```python
from build123d import *

# Parameters (mm, degrees)
SKETCH1_R               = 6.35
SKETCH1_W               = 19.05
SKETCH1_H               = 25.985863096
EXTRUDE2_DEPTH          = 14.3002
SKETCH2_W               = 19.05
SKETCH2_H               = 69.85
EXTRUDE3_DEPTH          = 23.8252
CUT_EXTRUDE1_DEPTH      = 73.599512703
CUT_EXTRUDE1_DEPTH_BACK = 73.599512703
CUT_EXTRUDE2_START      = -19.05
CUT_EXTRUDE2_DEPTH      = 19.05
EXTRUDE4_DEPTH          = 19.05
EXTRUDE4_DEPTH_BACK     = 38.1
FILLET1_R               = 6.35


# Read off the part's stored shape, not the designer's step: Cut-Extrude2
with BuildPart() as part:
    # Sketch1 → Extrude2 (new body)
    # profile 1 of 2: a face of its own
    with BuildSketch(Plane(origin=(0, 0, 0), x_dir=(1, 0, 0), z_dir=(0, 1, 0))):
        Polygon((-44.03422619, -11.566071429), (-44.03422619, 14.419791667), (-72.60922619, 14.419791667), (-72.60922619, -42.730208333), (3.59077381, -42.730208333), (3.59077381, 14.419791667), (-24.98422619, 14.419791667), (-24.98422619, -11.566071429), align=None)
        with Locations(Location((-56.73422619, -26.855208333, 0), (0, 0, 270))):
            Circle(SKETCH1_R, mode=Mode.SUBTRACT)
        with Locations(Location((-12.28422619, -26.855208333, 0), (0, 0, 270))):
            Circle(SKETCH1_R, mode=Mode.SUBTRACT)
    # profile 2 of 2: a face of its own
    with BuildSketch(Plane(origin=(0, 0, 0), x_dir=(1, 0, 0), z_dir=(0, 1, 0))):
        with Locations((-34.50922619, 1.426860119)):
            Rectangle(SKETCH1_W, SKETCH1_H)
    extrude(amount=-EXTRUDE2_DEPTH)

    # Sketch2 → Extrude3 (add)
    with BuildSketch(Plane(origin=(0, 0, 0), x_dir=(-1, 0, 0), z_dir=(0, 1, 0))):
        with Locations((34.50922619, -14.419791667)):
            Rectangle(SKETCH2_W, SKETCH2_H)
    extrude(amount=EXTRUDE3_DEPTH)

    # Sketch3 → Cut-Extrude1 (cut, two sides: drawn at the far end of the back side and taken through both)
    with BuildSketch(Plane.ZY.offset(44.03422619).offset(-CUT_EXTRUDE1_DEPTH_BACK)):
        Polygon((20.505208333, 23.8252), (-14.419791667, 23.8252), (20.505208333, 0), align=None)
    extrude(amount=CUT_EXTRUDE1_DEPTH + CUT_EXTRUDE1_DEPTH_BACK, mode=Mode.SUBTRACT)

    # Cut-Extrude2 outline → Cut-Extrude2 (cut)
    with BuildSketch(Plane.ZY.offset(44.03422619).offset(CUT_EXTRUDE2_START)):
        Polygon((-49.344791667, 0), (-14.419791667, 0), (-49.344791667, 23.8252), align=None)
    extrude(amount=CUT_EXTRUDE2_DEPTH, mode=Mode.SUBTRACT)

    # Sketch5 → Extrude4 (add, two sides: drawn at the far end of the back side and taken through both)
    with BuildSketch(Plane(origin=(-24.98422619, 0, -14.419791667), x_dir=(0, 0, -1), z_dir=(1, 0, 0)).offset(-EXTRUDE4_DEPTH_BACK)):
        Polygon((0, 23.8252), (0, 46.0502), (7.9502, 46.0502), (7.9502, 36.5252), (34.925, 36.5252), (34.925, 23.8252), align=None)
    extrude(amount=EXTRUDE4_DEPTH + EXTRUDE4_DEPTH_BACK)

    # Fillet1
    fillet1_edges = [part.edges().sort_by_distance(p)[0] for p in [
        (3.59077381, -7.1501, 42.730208333),
        (-72.60922619, -7.1501, 42.730208333),
        (-72.60922619, -7.1501, -14.419791667),
        (3.59077381, -7.1501, -14.419791667),
    ]]
    fillet(fillet1_edges, radius=FILLET1_R)


solid = part.part
```
Check sheet for the modelled part. Datum: model origin and axes. Units: mm. A direction names the side the tool comes from. Give positions to 0.01 mm unless a question says otherwise; leave off trailing zeros. Write each loop counter-clockwise with the first axis right and the second up, starting at its lowest first coordinate (ties: lowest second). Pieces come first, ordered by that corner, then holes. Notation, with made-up numbers: (-21.5, 70.5) - (-6.5, 70.5) arc R18 ccw to (-6.5, 84.5) - close; hole circle Ø5 at (37, -4). An arc over 180 degrees is marked (long way). Answer as a JSON object with one key per item and string values. Group by question number.
1) Sectioned sample at C-C (z = -42). Record the cut outline in (x, y), then the cut area to 3 significant figures.
2) Release check for a two-part mould opening along X. For faces 4 (the face through (1.68, -7.25, -12.61)), 5 (the face through (-35, 36.525, -36)), 6 (the face through (-63.084, 33, -28)), 7 (the face through (-16.15, -7.05, 21.82)) record: pulls with the +X half, pulls with the -X half, needs draft (parallel to the pull), parting line crosses it, or undercut.
3) Depth check by flat-ended pin: P1, Ø14.5, axis at x = -12.28, z = 26.86, coming from the -Y side; P2, Ø1.5, axis at x = -28.5, z = -12.5, coming from the +Y side; P3, Ø18, axis at y = 30, z = -33, coming from the +X side; P4, Ø6.5, axis at y = 35, z = -24.5, coming from the -X side. Enter the tip coordinate at first touch or a pass-through.
4) Sectioned sample at B-B (y = -3). Record the cut outline in (x, z), then the cut area to 3 significant figures.
5) Access from +Z, -Z, +X, -X, +Y, -Y to the whole of each face (thin tool, end or side, straight path). Record for faces 1 (the face through (-35, 41, -22.37)), 2 (the face through (-24.984, 12, -15)), 3 (the face through (-44.034, 12, -15)).
6) Thickness scan on probe 1 along Z at (x, y) = (-41.5, 32.5); probe 2 along Y at (x, z) = (-20, 37); probe 3 along Y at (x, z) = (-11, -28). Record the ranges inside material, lowest first. Write a range as from..to.
7) Sectioned sample at A-A (x = -47). Record the cut outline in (y, z).
8) Sectioned sample at D-D (x = -39). Record the cut outline in (y, z).
Geometry results:
{
 "1": {"outline": "(-63.08, 23.83) - (-44.03, 23.83) - (-44.03, 18.81) - (-24.98, 18.81) - (-24.98, 23.83) - (-5.93, 23.83) - (-5.93, 36.53) - (-63.08, 36.53) - close", "area": "821 mm^2"},
 "2": {"face 4": "pulls with the +X half", "face 5": "needs draft", "face 6": "pulls with the -X half", "face 7": "undercut"},
 "3": {"P1": "stops at y = -14.3", "P2": "stops at y = 23.03", "P3": "stops at x = -5.93", "P4": "stops at x = -63.08"},
 "4": {"outline": "(-72.61, -8.07) arc R6.35 ccw to (-66.26, -14.42) - (-2.76, -14.42) arc R6.35 ccw to (3.59, -8.07) - (3.59, 36.38) arc R6.35 ccw to (-2.76, 42.73) - (-66.26, 42.73) arc R6.35 ccw to (-72.61, 36.38) - close; hole circle Ø12.7 at (-56.73, 26.86); hole circle Ø12.7 at (-12.28, 26.86)", "area": "4,070 mm^2"},
 "5": {"face 1": "-Z, +X, -X, +Y", "face 2": "+Z, -Z, +X", "face 3": "+Z, -Z, -X"},
 "6": {"probe 1": "z = -49.34..-14.42", "probe 2": "y = -14.3..0", "probe 3": "y = 23.83..36.53"},
 "7": {"outline": "(-14.3, -14.42) - (0, -14.42) - (0, 42.73) - (-14.3, 42.73) - close; (23.83, -49.34) - (36.53, -49.34) - (36.53, -22.37) - (46.05, -22.37) - (46.05, -14.42) - (23.83, -14.42) - close"},
 "8": {"outline": "(-14.3, -14.42) - (0, -14.42) - (23.83, -49.34) - (36.53, -49.34) - (36.53, -22.37) - (46.05, -22.37) - (46.05, -14.42) - (23.83, -14.42) - (0, 20.51) - (0, 42.73) - (-14.3, 42.73) - close"}
}
